Check sheet for the modelled part. Datum: model origin and axes. Units: mm. A direction names the side the tool comes from. Round coordinates to 2 decimals unless told otherwise and drop trailing zeros. Order: outer loops, then holes, each group sorted by start corner. A loop starts at its lowest first (then second) coordinate and runs counter-clockwise, first axis right, second up. Notation, with made-up numbers: (34.5, 56.25) -> (93.5, 56.25) arc R28 cw to (93.5, 80.25) -> close; hole circle Ø2 at (-14.5, 12). An arc over 180 degrees is marked (long way). Use CSV: the item, a comma, the result in double quotes.
```python
from build123d import *

# Parameters (mm, degrees)
F0_R     = 25
F1_DEPTH = 50
F3_DEPTH = 50
F5_R     = 5
F6_DEPTH = 25


# Not quite as in the source:
# - after a boolean that leaves OpenCascade's solid faulty, fix() repairs it


with BuildPart() as f1:
    # F0 (on Top) → F1 (new body)
    with BuildSketch(Plane.XY):
        Circle(F0_R)
    extrude(amount=F1_DEPTH)

    # F2 (on face) → F3 (join)
    with BuildSketch(Plane.XY.offset(50)):
        with BuildLine():
            Line((23.8484800354, -7.5), (-23.8484800354, -7.5))
            ThreePointArc((-23.8484800354, -7.5), (0, -25), (23.8484800354, -7.5))
        make_face()
    extrude(amount=F3_DEPTH)

    # F4: F1 across plane


with BuildPart() as f1_1:
    add(f1.part)
    add(f1.part.mirror(Plane.XZ))

    add(f1_1.part.fix(), mode=Mode.REPLACE)

    # F5 (on Front) → F6 (cut, symmetric)
    with BuildSketch(Plane.XZ):
        with Locations((0, 75)):
            Circle(F5_R)
    extrude(amount=F6_DEPTH, both=True, mode=Mode.SUBTRACT)


solid = f1_1.part
```
Q1. Mould release check, pull along Z, two halves, no side actions. Record for faces 3 (the face through (-1.08, 16.13, 70.12)), 4 (the face through (0, -14, 100)), 5 (the face through (6, 7.5, 75)): pulls with the +Z half, pulls with the -Z half, needs draft (parallel to the pull), parting line crosses it, or undercut.
Result sheet:
face 3,"undercut"
face 4,"pulls with the +Z half"
face 5,"needs draft"
Q2. Sectioned sample at B-B, the plane z = 75. Enter the section's corners in (x, y).
Result sheet:
outline,"(-23.85, -7.5) arc R25 ccw to (-5, -24.49) -> (-5, -7.5) -> close; (-23.85, 7.5) -> (-5, 7.5) -> (-5, 24.49) arc R25 ccw to start; (5, -24.49) arc R25 ccw to (23.85, -7.5) -> (5, -7.5) -> close; (5, 7.5) -> (23.85, 7.5) arc R25 ccw to (5, 24.49) -> close"
Q3. Sectioned sample at A-A, the plane x = 0. Enter the section's corners in (y, z), then the cut area to 3 significant figures.
Result sheet:
outline,"(-25, 0) -> (25, 0) -> (25, 70) -> (7.5, 70) -> (7.5, 50) -> (-7.5, 50) -> (-7.5, 70) -> (-25, 70) -> close; (-25, 80) -> (-7.5, 80) -> (-7.5, 100) -> (-25, 100) -> close; (7.5, 80) -> (25, 80) -> (25, 100) -> (7.5, 100) -> close"
area,"3,900 mm^2"
Q4. Sectioned sample at C-C, the plane z = 87.5. Enter the section's corners in (x, y).
Result sheet:
outline,"(-23.85, -7.5) arc R25 ccw to (23.85, -7.5) -> close; (-23.85, 7.5) -> (23.85, 7.5) arc R25 ccw to start"
Q5. Scan lines: L1, parallel to Z at x = 0, y = -11; L2, parallel to Y at x = -7.5, z = 53; L3, parallel to Z at x = -1, y = -2. Record each from-to range of solid material in increasing order.
Result sheet:
L1,"z = 0 to 70, 80 to 100"
L2,"y = -23.85 to -7.5, 7.5 to 23.85"
L3,"z = 0 to 50"
Q6. Access from +Z, -Z, +X, -X, +Y, -Y to the whole of each face (thin tool, end or side, straight path). Record for faces 1 (the face through (0, 0, 0)), 2 (the face through (0, 0, 50)).
Result sheet:
face 1,"-Z, +X, -X, +Y, -Y"
face 2,"+Z, +X, -X"
Q7. Sectioned sample at D-D, the plane x = -12. Enter the section's corners in (y, z).
Result sheet:
outline,"(-21.93, 0) -> (21.93, 0) -> (21.93, 100) -> (7.5, 100) -> (7.5, 50) -> (-7.5, 50) -> (-7.5, 100) -> (-21.93, 100) -> close"
Q8. Go/stop test with flat-tipped pins: pin 1 (9 mm diameter, centred on x = 0, z = 75, fed in from -Y); pin 2 (1 mm diameter, centred on x = -17.5, z = 28.5, fed in from -Y); pin 3 (4 mm diameter, centred on y = 16, z = 64, fed in from -X); pin 4 (1 mm diameter, centred on x = -7.5, z = 11, fed in from -Y). Record where each tip stops, or that it passes through.
Result sheet:
pin 1,"passes through"
pin 2,"stops at y = -18.33"
pin 3,"stops at x = -20.71"
pin 4,"stops at y = -24"
